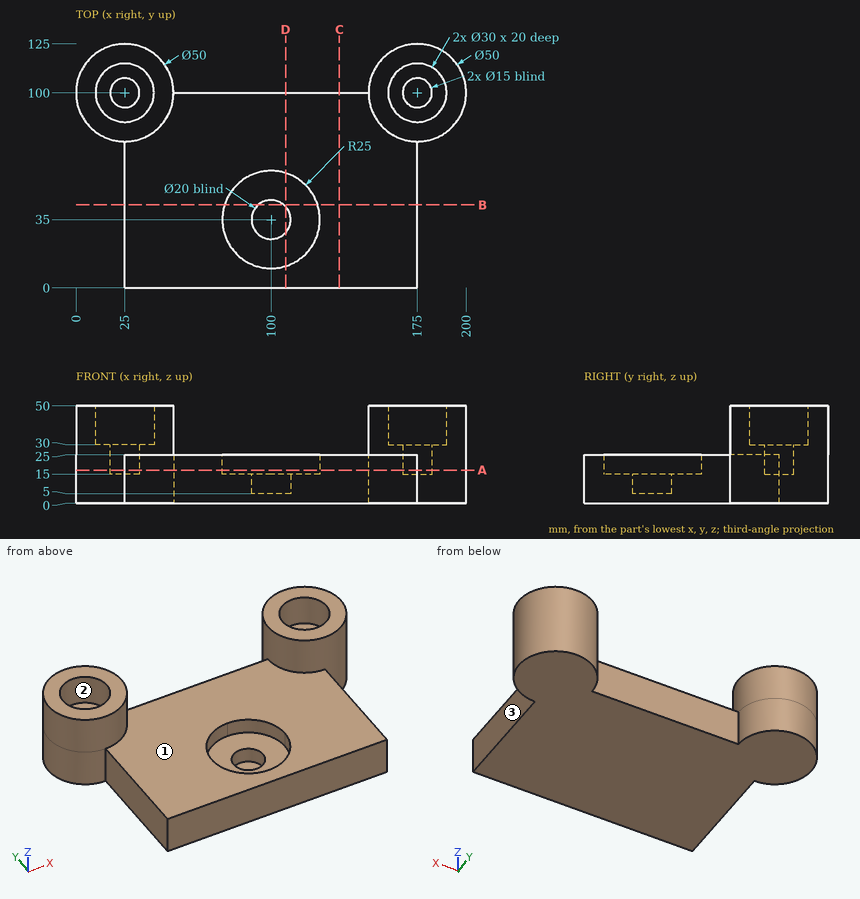
Here's the drawing with two shaded views (mm, measured from the low corner). I have some questions. A direction names the side the tool comes from. Give positions to 0.01 mm unless a question says otherwise; leave off trailing zeros. Write each loop counter-clockwise with the first axis right and the second up, starting at its lowest first coordinate (ties: lowest second). Pieces come first, ordered by that corner, then holes. Notation, with made-up numbers: (63.25, 48.5) - (83.25, 48.5) arc R33 cw to (83.25, 76.5) - close; hole circle Ø4 at (4.25, 19.25). An arc over 180 degrees is marked (long way). Write item = value, one per line. Start each with the question number.
1. Imagine slicing it at C-C (x = 135). Please give me the cut outline in (y, z).
2. Imagine slicing it at B-B (y = 42.5). Please give me the cut outline in (x, z).
3. Imagine slicing it at D-D (x = 107.5). Please give me the cut outline in (y, z), and give its area (3 significant figures).
4. On a 3-axis mill with a long thin cutter (end or side, diameter ignored), from which of +Z, -Z, +X, -X, +Y, -Y can I reach the whole of each face in a straight line? I mean the marked faces 1, 2 and 3. Say none if no direction works.
5. Please list where these lines run through material, in increasing order: line 1 (X direction, y = 100.5, z = 11) (3 decimals); line 2 (X direction, y = 94.5, z = 19); line 3 (Y direction, x = 175, z = 37.5).
6. Imagine slicing it at A-A (z = 17). Please give me the cut outline in (x, y), and give its area (3 significant figures).
7. For pin 1 (25 mm diameter, centred on x = 88, y = 25.5, fed in from +Z); pin 2 (16.5 mm diameter, centred on x = 24, y = 102, fed in from +Z); pin 3 (3 mm diameter, centred on y = 106, z = 16.5, fed in from +X), each with a flat end and sliding along its axis, tell me the tip position at first contact or that it passes through.
Worked answers:
q1.outline = (0, 0) - (100, 0) - (100, 25) - (0, 25) - close
q2.outline = (25, 0) - (175, 0) - (175, 25) - (123.85, 25) - (123.85, 15) - (106.61, 15) - (106.61, 5) - (93.39, 5) - (93.39, 15) - (76.15, 15) - (76.15, 25) - (25, 25) - close
q3.outline = (0, 0) - (100, 0) - (100, 25) - (58.85, 25) - (58.85, 15) - (41.61, 15) - (41.61, 5) - (28.39, 5) - (28.39, 15) - (11.15, 15) - (11.15, 25) - (0, 25) - close
q3.area = 1,890 mm2
q4.face_1 = +Z, -Y
q4.face_2 = +Z
q4.face_3 = +Z, -Z, +X, -Y
q5.line_1 = 0.005 to 49.995, 150.005 to 199.995
q5.line_2 = 0.61 to 19.9, 30.1 to 169.9, 180.1 to 199.39
q5.line_3 = 75 to 85, 115 to 125
q6.outline = (25, 0) - (175, 0) - (175, 75) arc R25 ccw (long way) to (150, 100) - (50, 100) arc R25 ccw (long way) to (25, 75) - close; hole circle Ø15 at (25, 100); hole circle Ø50 at (100, 35); hole circle Ø15 at (175, 100)
q6.area = 15,600 mm2
q7.pin_1 = 25
q7.pin_2 = 30
q7.pin_3 = 199.59
